Autodesk Inventor part; units mm, degrees
ref_plane "YZ Plane" through (0, 0, 0) normal (1, 0, 0) x (0, 1, 0)
ref_plane "XZ Plane" through (0, 0, 0) normal (0, 1, 0) x (-1, 0, 0)
ref_plane "XY Plane" through (0, 0, 0) normal (0, 0, 1) x (1, 0, 0)
sketch "Sketch5" plane through (0, 0, 0) normal (0, 1, 0) x (-1, 0, 0)
  line L0 (-12.8932, 28.65) -> (12.9, 28.65)
  line L1 (16.5, 25.05) -> (16.5, -25.0432)
  line L2 (12.8932, -28.65) -> (-12.8932, -28.65)
  line L3 (-16.5, -25.0432) -> (-16.5, 25.0432)
  line L4 (-16.5, 28.65) -> (16.5, -28.65) construction
  line L5 (16.5, 28.65) -> (-16.5, -28.65) construction
  arc A0 (16.5, 25.05) -> (12.9, 28.65) centre (12.9, 25.05) ccw
  line L6 (12.9, 28.65) -> (12.9, 25.05) construction
  line L7 (12.9, 25.05) -> (16.5, 25.05) construction
  arc A1 (12.8932, -28.65) -> (16.5, -25.0432) centre (12.8932, -25.0432) ccw
  arc A2 (-12.8932, 28.65) -> (-16.5, 25.0432) centre (-12.8932, 25.0432) ccw
  arc A3 (-16.5, -25.0432) -> (-12.8932, -28.65) centre (-12.8932, -25.0432) ccw
  circle A4 centre (13.5, 25.6528) radius 0.9915
  line L8 (11.2085, 27.55) -> (-11.2085, 27.55)
  arc A5 (-15.517, 25.05) -> (-15.517, 25.0432) centre (-12.8932, 25.0432) ccw
  line L9 (-15.4, 23.3613) -> (-15.4, -23.3613)
  line L10 (-11.2085, -27.55) -> (11.2085, -27.55)
  line L11 (15.4, -23.3613) -> (15.4, 23.3613)
  line L12 (12.5085, 25.6528) -> (12.5085, 26.25)
  line L13 (13.5, 24.6613) -> (14.1, 24.6613)
  arc A6 (12.5085, 26.25) -> (11.2085, 27.55) centre (11.2085, 26.25) ccw
  arc A7 (15.4, 23.3613) -> (14.1, 24.6613) centre (14.1, 23.3613) ccw
  line L14 (15.4, 0) -> (-15.4, 0) construction
  line L15 (0, 27.55) -> (0, -27.55) construction
  circle A8 centre (13.5, -25.6528) radius 0.9915
  line L16 (12.5085, -25.6528) -> (12.5085, -26.25)
  line L17 (13.5, -24.6613) -> (14.1, -24.6613)
  arc A9 (11.2085, -27.55) -> (12.5085, -26.25) centre (11.2085, -26.25) ccw
  arc A10 (14.1, -24.6613) -> (15.4, -23.3613) centre (14.1, -23.3613) ccw
  line L18 (0, -27.55) -> (0, 27.55) construction
  circle A11 centre (-13.5, 25.6528) radius 0.9915
  line L19 (-12.5085, 25.6528) -> (-12.5085, 26.25)
  line L20 (-13.5, 24.6613) -> (-14.1, 24.6613)
  arc A12 (-11.2085, 27.55) -> (-12.5085, 26.25) centre (-11.2085, 26.25) ccw
  arc A13 (-14.1, 24.6613) -> (-15.4, 23.3613) centre (-14.1, 23.3613) ccw
  arc A14 (-12.5085, -26.25) -> (-11.2085, -27.55) centre (-11.2085, -26.25) ccw
  line L21 (-12.5085, -25.6528) -> (-12.5085, -26.25)
  circle A15 centre (-13.5, -25.6528) radius 0.9915
  line L22 (-13.5, -24.6613) -> (-14.1, -24.6613)
  arc A16 (-15.4, -23.3613) -> (-14.1, -24.6613) centre (-14.1, -23.3613) ccw
  line L23 (-12.1355, -25.3386) -> (-12.1355, -25.333)
  line L24 (14.7139, 22.2154) -> (14.827, 22.0092) construction
  circle A17 centre (0, 12.583) radius 7.25
  arc A18 (6.3593, 25.2794) -> (-6.3593, 25.2794) centre (0, 12.583) ccw
  arc A19 (-6.3593, -0.1134) -> (6.3593, -0.1134) centre (0, 12.583) ccw
  line L25 (0, 12.583) -> (-6.3593, -0.1134) construction
  line L26 (0, 12.583) -> (6.3593, -0.1134) construction
  line L27 (0, 12.583) -> (0, -1.617) construction
  line L28 (0, 12.583) -> (16.5, 12.583) construction
  line L29 (-6.3593, -0.1134) -> (-6.3593, 25.2794) construction
  line L30 (6.3593, -0.1134) -> (6.3593, 25.2794) construction
  arc A20 (-6.3593, -0.1134) -> (-6.9877, -0.2666) centre (-6.5832, -0.5605) ccw
  line L31 (-6.9877, -0.2666) -> (-6.5832, -0.5605) construction
  line L32 (-6.5832, -0.5605) -> (-6.3593, -0.1134) construction
  line L33 (-6.9877, -0.2666) -> (-7.2816, -0.671)
  arc A21 (-10.5175, 1.6804) -> (-7.2816, -0.671) centre (-8.8995, 0.5047) ccw
  line L34 (-10.5175, 1.6804) -> (-10.2236, 2.0849)
  arc A22 (-10.2236, 2.0849) -> (-10.2728, 2.7402) centre (-10.6345, 2.3835) ccw
  line L35 (-10.2236, 2.0849) -> (-10.6345, 2.3835) construction
  line L36 (-10.6345, 2.3835) -> (-10.2728, 2.7402) construction
  arc A23 (6.9877, -0.2666) -> (6.3593, -0.1134) centre (6.5832, -0.5605) ccw
  line L37 (6.9877, -0.2666) -> (7.2816, -0.671)
  arc A24 (7.2816, -0.671) -> (10.5175, 1.6804) centre (8.8995, 0.5047) ccw
  line L38 (10.5175, 1.6804) -> (10.2236, 2.0849)
  arc A25 (10.2728, 2.7402) -> (10.2236, 2.0849) centre (10.6345, 2.3835) ccw
  arc A26 (-6.9877, 25.4326) -> (-6.3593, 25.2794) centre (-6.5832, 25.7265) ccw
  line L39 (-6.9877, 25.4326) -> (-7.2816, 25.837)
  arc A27 (-7.2816, 25.837) -> (-10.5175, 23.4856) centre (-8.8995, 24.6613) ccw
  line L40 (-10.5175, 23.4856) -> (-10.2236, 23.0811)
  arc A28 (-10.2728, 22.4258) -> (-10.2236, 23.0811) centre (-10.6345, 22.7825) ccw
  arc A29 (6.3593, 25.2794) -> (6.9877, 25.4326) centre (6.5832, 25.7265) ccw
  line L41 (6.9877, 25.4326) -> (7.2816, 25.837)
  arc A30 (10.5175, 23.4856) -> (7.2816, 25.837) centre (8.8995, 24.6613) ccw
  line L42 (10.5175, 23.4856) -> (10.2236, 23.0811)
  arc A31 (10.2236, 23.0811) -> (10.2728, 22.4258) centre (10.6345, 22.7825) ccw
  arc A32 (-10.2728, 22.4258) -> (-10.2728, 2.7402) centre (0, 12.583) ccw
  arc A33 (10.2728, 2.7402) -> (10.2728, 22.4258) centre (0, 12.583) ccw
  circle A34 centre (0, -12.96) radius 3.955
  line L43 (0, -12.96) -> (0, -18.96) construction
  circle A35 centre (13.5, -25.6528) radius 2
  line L44 (13.5, -25.6528) -> (13.5, -23.6528) construction
  line L45 (13.5, -25.6528) -> (11.5, -25.6528) construction
  line L46 (13.5, -23.6528) -> (15.3669, -23.6528) construction
  line L47 (11.5, -25.6528) -> (11.5, -27.5169) construction
  circle A36 centre (-13.5, -25.6528) radius 2
  circle A37 centre (-13.5, 25.6528) radius 2
  circle A38 centre (13.5, 25.6528) radius 2
  circle A39 centre (0, -12.843) radius 4.5212
  circle A40 centre (0, -14.56) radius 6.25
  line L48 (0, -14.56) -> (-5.807, -24.618) construction
  line L49 (0, -14.56) -> (5.807, -24.618) construction
  arc A41 (-4.057, -21.5869) -> (4.057, -21.5869) centre (0, -14.56) ccw
  arc A42 (-4.057, -21.5869) -> (-6.3593, -22.0899) centre (-4.932, -23.1025) ccw
  arc A43 (6.3306, -22.0506) -> (4.057, -21.5869) centre (4.932, -23.1025) ccw
  line L50 (0, -26.174) -> (-8.43, -26.174)
  line L51 (0, -26.174) -> (8.4301, -26.174)
  line L52 (8.8297, -25.3735) -> (6.3306, -22.0506)
  arc A44 (8.4301, -26.174) -> (8.8297, -25.3735) centre (8.4301, -25.674) ccw
  line L53 (-8.8295, -25.3734) -> (-6.3593, -22.0899)
  arc A45 (-8.8295, -25.3734) -> (-8.43, -26.174) centre (-8.43, -25.674) ccw
  line L54 (-4.8269, -4.2707) -> (-13.3585, -4.2707)
  line L55 (-13.8585, -4.7707) -> (-13.8585, -20.2911)
  line L56 (-12.9875, -20.6263) -> (-8.5656, -15.7334)
  arc A46 (-13.8585, -20.2911) -> (-12.9875, -20.6263) centre (-13.3585, -20.2911) ccw
  arc A47 (-13.3585, -4.2707) -> (-13.8585, -4.7707) centre (-13.3585, -4.7707) ccw
  line L57 (5.0371, -4.2707) -> (13.3585, -4.2707)
  line L58 (13.8585, -4.7707) -> (13.8585, -20.2921)
  line L59 (12.9875, -20.6273) -> (8.5655, -15.7332)
  arc A48 (12.9875, -20.6273) -> (13.8585, -20.2921) centre (13.3585, -20.2921) ccw
  arc A49 (13.8585, -4.7707) -> (13.3585, -4.2707) centre (13.3585, -4.7707) ccw
  arc A50 (8.114, -14.56) -> (4.057, -7.5331) centre (0, -14.56) ccw
  arc A51 (-4.057, -7.5331) -> (-8.114, -14.56) centre (0, -14.56) ccw
  arc A52 (8.114, -14.56) -> (8.5655, -15.7332) centre (9.864, -14.56) ccw
  arc A53 (5.0371, -4.2707) -> (4.057, -7.5331) centre (5.0371, -6.0491) ccw
  arc A54 (-4.057, -7.5331) -> (-4.8269, -4.2707) centre (-4.8269, -5.9927) ccw
  arc A55 (-8.5656, -15.7334) -> (-8.114, -14.56) centre (-9.864, -14.56) ccw
  line L60 (10.7841, 22.7925) -> (11.0216, 23.1193)
  arc A56 (11.0216, 23.1193) -> (6.7775, 26.2034) centre (8.8995, 24.6613) ccw
  line L61 (6.7775, 26.2034) -> (6.5448, 25.883)
  arc A57 (6.5448, 25.883) -> (-6.5448, 25.883) centre (0, 12.583) ccw
  line L62 (-6.5448, 25.883) -> (-6.7775, 26.2034)
  arc A58 (-6.7775, 26.2034) -> (-11.0216, 23.1193) centre (-8.8995, 24.6613) ccw
  line L63 (-11.0216, 23.1193) -> (-10.7841, 22.7925)
  arc A59 (-10.7841, 22.7925) -> (-10.7841, 2.3735) centre (0, 12.583) ccw
  line L64 (-10.7841, 2.3735) -> (-11.0216, 2.0467)
  arc A60 (-11.0216, 2.0467) -> (-6.7775, -1.0374) centre (-8.8995, 0.5047) ccw
  line L65 (-6.7775, -1.0374) -> (-6.5448, -0.717)
  arc A61 (-6.5448, -0.717) -> (6.5448, -0.717) centre (0, 12.583) ccw
  line L66 (6.5448, -0.717) -> (6.7775, -1.0374)
  arc A62 (6.7775, -1.0374) -> (11.0216, 2.0467) centre (8.8995, 0.5047) ccw
  line L67 (11.0216, 2.0467) -> (10.7841, 2.3735)
  arc A63 (10.7841, 2.3735) -> (10.7841, 22.7925) centre (0, 12.583) ccw
  point P0 (0, 0)
  point P1 (0, 0)
  point P2 (-2.4, 0)
  point P3 (-12.1591, 27.1367)
  point P4 (-14.9852, 24.3133)
  point P5 (-14.9852, -24.3133)
  point P6 (-12.1591, -27.1367)
  point P7 (12.1591, -27.1367)
  point P8 (14.9852, -24.3133)
  point P9 (14.9852, 24.3133)
  point P10 (12.1591, 27.1367)
  point P11 (5.807, -24.501)
  point P12 (13.8585, -4.2707)
  dimension "d61" = 57.3
  dimension "d62" = 33
  dimension "d63" = 3.6
  dimension "d64" = 90
  dimension "d65" = 3.6068
  dimension "d66" = 3.6068
  dimension "d67" = 2.9972
  dimension "d68" = 3
  dimension "d69" = 1.983
  dimension "d70" = 1.1
  dimension "d71" = 1.3
  dimension "d74" = 22.417
  dimension "d84" = 14.5
  dimension "d85" = 28.4
  dimension "d87" = 53.21
  dimension "d88" = 0.5
  dimension "d89" = 80.6
  dimension "d90" = 0.5
  dimension "d91" = 2
  dimension "d92" = 0.508
  dimension "d93" = 80.6
  dimension "d98" = 25.543
  dimension "d99" = 7.91
  dimension "d116" = 4
  dimension "d117" = 4
  dimension "d118" = 4
  dimension "d119" = 4
  dimension "d128" = 9.0424
  dimension "d129" = 1.6
  dimension "d130" = 12.5
  dimension "d131" = 60
  dimension "d132" = 30
  dimension "d145" = 0.5
  dimension "d146" = 0.5
  dimension "d147" = 0.5
  dimension "d148" = 0.5
  dimension "d151" = 360
  dimension "d192" = 1.1
  dimension "d193" = 1.1
  dimension "d195" = 1.1
extrude "Extrusion6" add sketch "Sketch5" against normal blind 13.5 contours L0 A0 L1 A1 L2 A3 L3 A2 | A4 | A4 L12 A6 A38 A7 L13 | A4 L13 A7 A38 A6 L12 | A38 A7 L11 A10 A35 A9 L10 A14 A36 A16 L9 A13 A37 A12 L8 A6 | A37 A13 L20 A11 L19 A12 | A12 L19 A11 L20 A13 A37 | A35 A9 L16 A8 L17 A10 | A10 L17 A8 L16 A9 A35 | A11 | A8 | A36 A14 L21 A15 L22 A16 | A16 L22 A15 L21 A14 A36 | A15 | A29 L41 A30 L42 A31 A33 A25 L38 A24 L37 A23 A19 A20 L33 A21 L34 A22 A32 A28 L40 A27 L39 A26 A18 | A34 | A39 | A40 | A41 A43 L52 A44 L51 L50 A45 L53 A42 | A54 A51 A55 L56 A46 L55 A47 L54 | L57 A49 L58 A48 L59 A52 A50 A53 | A63 L67 A62 L66 A61 L65 A60 L64 A59 L63 A58 L62 A57 L61 A56 L60
extrude "Extrusion9" cut sketch "Sketch5" against normal blind 22 contours A4 L13 A7 A38 A6 L12 | A38 A7 L11 A10 A35 A9 L10 A14 A36 A16 L9 A13 A37 A12 L8 A6 | A37 A13 L20 A11 L19 A12 | A10 L17 A8 L16 A9 A35 | A36 A14 L21 A15 L22 A16 | A29 L41 A30 L42 A31 A33 A25 L38 A24 L37 A23 A19 A20 L33 A21 L34 A22 A32 A28 L40 A27 L39 A26 A18 | A34 | A39 | A40 | A41 A43 L52 A44 L51 L50 A45 L53 A42 | A54 A51 A55 L56 A46 L55 A47 L54 | L57 A49 L58 A48 L59 A52 A50 A53 | A63 L67 A62 L66 A61 L65 A60 L64 A59 L63 A58 L62 A57 L61 A56 L60 picked at (13.7589, 24.3277) picked at (-13.7763, 24.3295) picked at (13.7589, -24.3277) picked at (-13.7763, -24.3295)
extrude "Extrusion10" add sketch "Sketch5" against normal blind 12.5 contours A4 L13 A7 A38 A6 L12 | A37 A13 L20 A11 L19 A12 | A10 L17 A8 L16 A9 A35 | A36 A14 L21 A15 L22 A16 picked at (13.7589, 24.3277) picked at (-13.7763, 24.3295) picked at (13.7589, -24.3277) picked at (-13.7763, -24.3295)
extrude "Extrusion11" add sketch "Sketch5" against normal blind 11.5 contours A34 | A39 | A40
extrude "Extrusion12" cut sketch "Sketch5" against normal blind 11.5 contours A34 | A39
extrude "Extrusion13" add sketch "Sketch5" against normal blind 12.5 contours A38 A7 L11 A10 A35 A9 L10 A14 A36 A16 L9 A13 A37 A12 L8 A6
extrude "Extrusion14" add sketch "Sketch5" along normal blind 1.5 contours L0 A0 L1 A1 L2 A3 L3 A2 | A4 | A4 L12 A6 A38 A7 L13 | A4 L13 A7 A38 A6 L12 | A38 A7 L11 A10 A35 A9 L10 A14 A36 A16 L9 A13 A37 A12 L8 A6 | A37 A13 L20 A11 L19 A12 | A12 L19 A11 L20 A13 A37 | A35 A9 L16 A8 L17 A10 | A10 L17 A8 L16 A9 A35 | A11 | A8 | A36 A14 L21 A15 L22 A16 | A16 L22 A15 L21 A14 A36 | A15 | A29 L41 A30 L42 A31 A33 A25 L38 A24 L37 A23 A19 A20 L33 A21 L34 A22 A32 A28 L40 A27 L39 A26 A18 | A40 | A63 L67 A62 L66 A61 L65 A60 L64 A59 L63 A58 L62 A57 L61 A56 L60
sketch "Sketch13" plane through (0, 0, 0) normal (0, -1, 0) x (1, 0, 0)
  arc A0 (-6.5448, -0.717) -> (6.5448, -0.717) centre (0, 12.583) ccw construction
  line L0 (0, -2.2401) -> (0, 1.5699) construction
  arc A1 (1.048, -2.203) -> (-1.048, -2.203) centre (0, -0.4621) ccw
  arc A2 (-1.048, -2.203) -> (1.048, -2.203) centre (0, 12.583) ccw
  line L1 (1.5178, -2.1622) -> (1.8929, -1.2009)
  line L2 (-1.8929, -1.2009) -> (-1.5178, -2.1622)
  arc A3 (-1.5178, -2.1622) -> (1.5178, -2.1622) centre (0, 12.583) ccw
  point P0 (0, 0)
  point P1 (-1.048, -2.203)
  point P2 (1.048, -2.203)
  dimension "d204" = 3.81
  dimension "d205" = 2.032
extrude "Extrusion22" add sketch "Sketch13" along normal blind 1.5
properties part number "CapOGStyle" material "Plastic, Opaque Black"
Work out the finished part from the listing and answer in its coordinate system (mm). A direction names the side the tool comes from. Give positions to 0.01 mm unless a question says otherwise; leave off trailing zeros. Order: outer loops, then holes, each group sorted by start corner. A loop starts at its lowest first (then second) coordinate and runs counter-clockwise, first axis right, second up. Notation, with made-up numbers: (26, -38) - (62, -38) arc R18 ccw to (62, -15) - close; hole circle Ø5 at (29.5, 15). An arc over 180 degrees is marked (long way). Answer as CSV lines item,"result". Start each with the question number.
Q1. The part is cut by section C-C (z = -12). Write down the section's boundary in (x, y), then the cut area to 3 significant figures.
Q2. The part is cut by section B-B (z = -24). Write down the section's boundary in (x, y).
Q3. The mould has two halves that part along X. Classify faces 1 (the face through (9, -5, -4.271)), 2 (the face through (0, -6, -28.65)), 3 (the face through (15.471, -6.105, 27.565)): +X half, -X half, draft (parallel to the pull), parting line (faces both ways), or undercut.
Q4. For faces 4 (the face through (7.61, -5.4, -23.75)), 5 (the face through (12.118, -12.993, 27.179)), 6 (the face through (-15.42, -6.1, 27.62)), determine the directions among +Z, -Z, +X, -X, +Y, -Y from which every point of the face is accessible in a straight line to the end or side of a thin tool.
Q5. Given pin 1 Ø2 at (x, z) = (-4, -11) entering from -Y; pin 2 Ø13 at (x, z) = (0, 12.583) entering from +Y; pin 3 Ø0.5 at (y, z) = (-13, 26) entering from +X; pin 4 Ø6 at (x, z) = (1.5, -14.5) entering from -Y, each flat-ended and moving along its own axis, determine where each tip first touches the part or whether it passes through.
Q6. The part is cut by section A-A (x = 0). Give the number of separate pieces and of enclosed holes in the cut face, then the cut area to 3 significant figures.
Q7. Find the intervals of material crossed by L1, parallel to Z at x = 0, y = -12.05; L2, parallel to Z at x = -2.5, y = -9; L3, parallel to Z at x = -10, y = -8.5, in increasing order. Write a range as [from, to].
Check result:
1,outline,"(-16.5, -13.5) - (-15.4, -13.5) - (-15.4, -12.5) - (-13.86, -12.5) - (-13.86, 1.5) - (-16.5, 1.5) - close; (-7.7, -12.5) - (-5.7, -12.5) - (-5.7, -11.5) - (-4.44, -11.5) - (-4.44, 1.5) - (-7.7, 1.5) - close; (4.44, -11.5) - (5.7, -11.5) - (5.7, -12.5) - (7.7, -12.5) - (7.7, 1.5) - (4.44, 1.5) - close; (13.86, -12.5) - (15.4, -12.5) - (15.4, -13.5) - (16.5, -13.5) - (16.5, 1.5) - (13.86, 1.5) - close"
1,area,"165 mm²"
2,outline,"(-16.5, -13.5) - (-15.23, -13.5) - (-15.23, -12.5) - (-7.8, -12.5) - (-7.8, 1.5) - (-16.5, 1.5) - close; (7.8, -12.5) - (15.23, -12.5) - (15.23, -13.5) - (16.5, -13.5) - (16.5, 1.5) - (7.8, 1.5) - close"
3,face 1,"undercut"
3,face 2,"draft"
3,face 3,"+X half"
4,face 4,"+Y, -Y"
4,face 5,"-Y"
4,face 6,"+Z, -X, +Y, -Y"
5,pin 1,"stops at y = -12.5"
5,pin 2,"passes through"
5,pin 3,"stops at x = 16.43"
5,pin 4,"stops at y = -11.5"
6,separate pieces,"4"
6,enclosed holes,"0"
6,area,"239 mm²"
7,L1,"z = [-28.65, -26.17], [-22.67, -20.81], [-8.31, -2.24], [27.41, 28.65]"
7,L2,"z = [-28.65, -26.17], [-22.28, -16.61], [-9.08, -2.03], [27.19, 28.65]"
7,L3,"z = [-28.65, -17.32], [-4.27, -1.88], [27.04, 28.65]"
